The model under review builds one solid part; all positions refer to its coordinate system, in mm. A direction names the side the tool comes from. Round coordinates to 2 decimals unless told otherwise and drop trailing zeros. Write each loop counter-clockwise with the first axis right and the second up, starting at its lowest first coordinate (ties: lowest second). Pieces come first, ordered by that corner, then holes. Notation, with made-up numbers: (56.5, -25.5) -> (95.5, -25.5) arc R11 cw to (95.5, -10.5) -> close; hole circle Ø9 at (-16.5, 37). An arc over 180 degrees is marked (long way). Return JSON: item names as keys, results as strings. Group by question number.
1. Take a section at C-C, the plane y = 35. Write out the cut boundary in (x, z).
2. Clearance check with flat-ended pins moving along their axes: P1, Ø10, axis at x = 139, y = 35, coming from the +Z side; P2, Ø4, axis at y = 19.5, z = 60.5, coming from the +X side; P3, Ø5, axis at y = 44, z = 39.5, coming from the +X side. State where each tip first meets the part, or that it passes through.
3. Mouldability with a two-part tool opening along Z and no side actions: class faces 4 (the flat face through (0, 35, 15)), 5 (the cylindrical face through (312, 29, 45)), 6 (the flat face through (320, 35, 70)) as pulls with the +Z half, pulls with the -Z half, needs draft (parallel to the pull), parting line crosses it, or undercut.
4. Take a section at B-B, the plane x = 320. Write out the cut boundary in (y, z), then the cut area to 3 significant figures.
5. Take a section at D-D, the plane z = 52.5. Write out the cut boundary in (x, y).
6. Tool access review of faces 1 (the cylindrical face through (301.525, 42.66, 64.93)), 2 (the flat face through (173, 0, 15)), 3 (the flat face through (315, 44, 60)): name each direction out of +Z, -Z, +X, -X, +Y, -Y from which nothing blocks a thin tool from reaching the whole face with its end or side.
7. For line 1 along Z through (x, y) = (326, 26.5); line 2 along Z through (x, y) = (94, 33); line 3 along X through (y, z) = (30.5, 46), list the stretches that pass through material, from the lowest coordinate up. Write a range as from..to.
8. Take a section at A-A, the plane y = 22. Write out the cut boundary in (x, z).
from build123d import *

# Parameters (mm, degrees)
CROQUIS1_W              = 350
CROQUIS1_H              = 70
SALIENTE_EXTRUIR1_DEPTH = 30
CROQUIS2_R              = 20
SALIENTE_EXTRUIR2_DEPTH = 40
CROQUIS4_R              = 20
CROQUIS4_R_2            = 10
CORTAR_EXTRUIR1_DEPTH   = 30


with BuildPart() as part:
    # Croquis1 → Saliente-Extruir1 (new body)
    with BuildSketch(Plane.XY):
        with Locations((175, 35)):
            Rectangle(CROQUIS1_W, CROQUIS1_H)
    extrude(amount=SALIENTE_EXTRUIR1_DEPTH)

    # Croquis2 → Saliente-Extruir2 (add)
    with BuildSketch(Plane.XY.offset(30)):
        with Locations(Location((320, 35, 0), (0, 0, 180))):
            Circle(CROQUIS2_R)
    extrude(amount=SALIENTE_EXTRUIR2_DEPTH)

    # Croquis4 → Cortar-Extruir1 (cut)
    with BuildSketch(Plane.XY.offset(30)):
        with Locations((320, 35)):
            Circle(CROQUIS4_R)
        with Locations((320, 35)):
            Circle(CROQUIS4_R_2, mode=Mode.SUBTRACT)
    extrude(amount=CORTAR_EXTRUIR1_DEPTH, mode=Mode.SUBTRACT)


solid = part.part
Output:
{
 "1": {"outline": "(0, 0) -> (350, 0) -> (350, 30) -> (330, 30) -> (330, 60) -> (340, 60) -> (340, 70) -> (300, 70) -> (300, 60) -> (310, 60) -> (310, 30) -> (0, 30) -> close"},
 "2": {"P1": "stops at z = 30", "P2": "stops at x = 334.76", "P3": "stops at x = 327.6"},
 "3": {"face 4": "needs draft", "face 5": "undercut", "face 6": "pulls with the +Z half"},
 "4": {"outline": "(0, 0) -> (70, 0) -> (70, 30) -> (45, 30) -> (45, 60) -> (55, 60) -> (55, 70) -> (15, 70) -> (15, 60) -> (25, 60) -> (25, 30) -> (0, 30) -> close", "area": "3,100 mm^2"},
 "5": {"outline": "circle Ø20 at (320, 35)"},
 "6": {"face 1": "+Z", "face 2": "+Z, -Z, +X, -X, -Y", "face 3": "none"},
 "7": {"line 1": "z = 0..30, 60..70", "line 2": "z = 0..30", "line 3": "x = 311.07..328.93"},
 "8": {"outline": "(0, 0) -> (350, 0) -> (350, 30) -> (0, 30) -> close; (304.8, 60) -> (335.2, 60) -> (335.2, 70) -> (304.8, 70) -> close"}
}
